from build123d import *

# Parameters (mm, degrees)
F1_DEPTH = 11.1125
F2_T     = -1.5875
F3_R     = 0.79375


with BuildPart() as f1:
    # F0 (on Right) → F1 (new body)
    with BuildSketch(Plane.YZ):
        Polygon((15.306922, -42.509722), (-3.743078, -42.509722), (-3.743078, -48.859722), (2.606922, -55.209722), (8.956922, -55.209722), (15.306922, -48.859722), align=None)
    extrude(amount=F1_DEPTH)

    # F2
    f2_openings = [f1.faces().sort_by_distance(p)[0] for p in [
        (5.55625, 5.781922, -42.509722),
    ]]
    offset(amount=F2_T, openings=f2_openings)

    # F3
    f3_edges = [f1.edges().sort_by_distance(p)[0] for p in [
        (11.1125, 5.781922, -42.509722),
        (11.1125, -3.743078, -45.684722),
        (11.1125, -0.568078, -52.034722),
        (11.1125, 5.781922, -55.209722),
        (11.1125, 12.131922, -52.034722),
        (11.1125, 15.306922, -45.684722),
        (0, 5.781922, -42.509722),
        (0, -3.743078, -45.684722),
        (0, -0.568078, -52.034722),
        (0, 5.781922, -55.209722),
        (0, 12.131922, -52.034722),
        (0, 15.306922, -45.684722),
    ]]
    fillet(f3_edges, radius=F3_R)


solid = f1.part
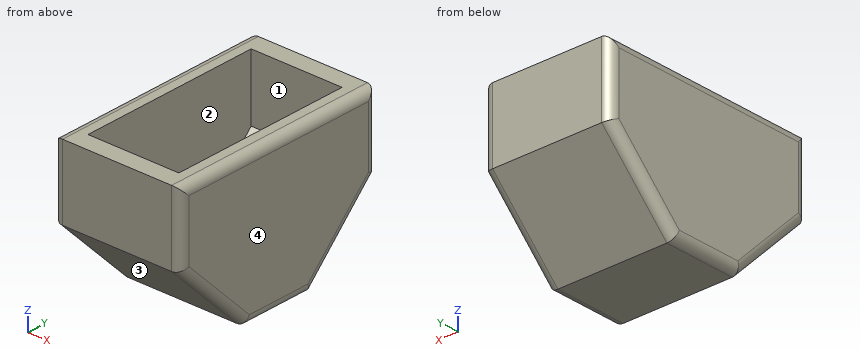
Here's how the part is built. I have some questions about the finished solid (model axes, mm). Face numbers are marked on the shaded views. Coordinates: 2 decimals unless noted, no trailing zeros. Order: outer loops, then holes, each group sorted by start corner. A loop starts at its lowest first (then second) coordinate and runs counter-clockwise, first axis right, second up. Notation, with made-up numbers: (-27.5, 34.25) -> (-11.5, 34.25) arc R15 ccw to (-11.5, 40.25) -> close; hole circle Ø2 at (24.5, -3.5). An arc over 180 degrees is marked (long way). Answer in a Markdown table with one row per item.
(1) I want a section at D-D on x = 1.25. List the corners of the cut face in (y, z) for me.
Answer key:
| item | result |
|---|---|
| outline | (-3.74, -48.86) -> (2.61, -55.21) -> (8.96, -55.21) -> (15.31, -48.86) -> (15.31, -42.51) -> (-3.74, -42.51) -> close |
(2) Thinking about a two-plate mould opening in X: for the marked faces 1, 2, 3 and 4, which applies, +X half, -X half, draft (parallel to the pull), parting line (faces both ways), or undercut?
Answer key:
| item | result |
|---|---|
| face 1 | undercut |
| face 2 | undercut |
| face 3 | draft |
| face 4 | +X half |
(3) I want a section at B-B on y = 7.75. List the corners of the cut face in (x, z) for me (1 decimal).
Answer key:
| item | result |
|---|---|
| outline | (0, -54.4) arc R0.8 ccw to (0.8, -55.2) -> (10.3, -55.2) arc R0.8 ccw to (11.1, -54.4) -> (11.1, -43.3) arc R0.8 ccw to (10.3, -42.5) -> (9.5, -42.5) -> (9.5, -53.6) -> (1.6, -53.6) -> (1.6, -42.5) -> (0.8, -42.5) arc R0.8 ccw to (0, -43.3) -> close |
(4) Please list where these lines run through material, in increasing order: probe 1 along Y at (x, z) = (4.75, -44.25); probe 2 along X at (y, z) = (7, -44) (1 decimal); probe 3 along Y at (x, z) = (0.75, -44).
Answer key:
| item | result |
|---|---|
| probe 1 | -3.74 to -2.16, 13.72 to 15.31 |
| probe 2 | 0 to 1.6, 9.5 to 11.1 |
| probe 3 | -3.74 to 15.31 |
(5) I want a section at A-A on z = -46.25. List the corners of the cut face in (x, y) for me (1 decimal).
Answer key:
| item | result |
|---|---|
| outline | (0, -2.9) arc R0.8 ccw to (0.8, -3.7) -> (10.3, -3.7) arc R0.8 ccw to (11.1, -2.9) -> (11.1, 14.5) arc R0.8 ccw to (10.3, 15.3) -> (0.8, 15.3) arc R0.8 ccw to (0, 14.5) -> close; hole (1.6, -2.2) -> (9.5, -2.2) -> (9.5, 13.7) -> (1.6, 13.7) -> close |
(6) I want a section at C-C on x = 7.75. List the corners of the cut face in (y, z) for me, then the cut area to 3 significant figures.
Answer key:
| item | result |
|---|---|
| outline | (-3.74, -48.86) -> (2.61, -55.21) -> (8.96, -55.21) -> (15.31, -48.86) -> (15.31, -42.51) -> (13.72, -42.51) -> (13.72, -48.2) -> (8.3, -53.62) -> (3.26, -53.62) -> (-2.16, -48.2) -> (-2.16, -42.51) -> (-3.74, -42.51) -> close |
| area | 54.6 mm^2 |
(7) Will these pins go through, and if not, where does the flat tip stop? pin 1 Ø6 at (x, y) = (9.5, 13) entering from -Z; pin 2 Ø1.5 at (x, y) = (7, 6) entering from +Z; pin 3 Ø4 at (x, y) = (5, 9.5) entering from +Z.
Answer key:
| item | result |
|---|---|
| pin 1 | z = -54.17 |
| pin 2 | z = -53.62 |
| pin 3 | z = -50.42 |
